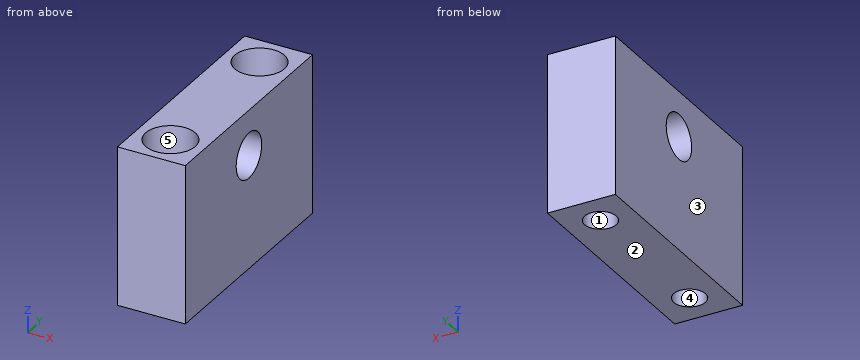
```python
from build123d import *

# Parameters (mm, degrees)
F0_W     = 15
F0_H     = 50
F1_DEPTH = 35
F2_R     = 5
F3_DEPTH = 15
F4_R     = 3.5
F5_DEPTH = 35
F6_R     = 5.5
F7_DEPTH = 9.5


with BuildPart() as f1:
    # F0 (on Top) → F1 (new body)
    with BuildSketch(Plane.XY):
        Rectangle(F0_W, F0_H)
    extrude(amount=F1_DEPTH)

    # F2 (on face) → F3 (cut, through all)
    with BuildSketch(Plane.YZ.offset(7.5)):
        with Locations((0, 25)):
            Circle(F2_R)
    extrude(amount=-F3_DEPTH, mode=Mode.SUBTRACT)

    # F4 (on face) → F5 (cut, through all)
    with BuildSketch(Plane.XY.offset(35)):
        with Locations((0, -17.5)):
            Circle(F4_R)
        with Locations((0, 17.5)):
            Circle(F4_R)
    extrude(amount=-F5_DEPTH, mode=Mode.SUBTRACT)

    # F6 (on face) → F7 (cut)
    with BuildSketch(Plane.XY.offset(35)):
        with Locations((0, -17.5)):
            Circle(F6_R)
        with Locations((0, 17.5)):
            Circle(F6_R)
    extrude(amount=-F7_DEPTH, mode=Mode.SUBTRACT)


solid = f1.part
```
The listing builds one solid part. Answer for the finished solid, in the listing's coordinates (mm). Face numbers are marked on the shaded views. A direction names the side the tool comes from. Round coordinates to 2 decimals unless told otherwise and drop trailing zeros. Loops run counter-clockwise (first coordinate to the right, second up) from the corner with the lowest first, then second, coordinate; pieces in that order, holes last.
1) Given P1, Ø3, axis at y = 2.5, z = 26, coming from the -X side, flat-ended and moving along its own axis, determine where the tip first touches the part or whether it passes through.
Outcome:
P1: passes through
2) A cutting plane is placed at D-D on x = -2.25. Determine the outline of the cut face in (y, z), plus the area to 3 significant figures.
Outcome:
outline: (-25, 0) - (-20.18, 0) - (-20.18, 25.5) - (-22.52, 25.5) - (-22.52, 35) - (-25, 35) - close; (-14.82, 0) - (14.82, 0) - (14.82, 25.5) - (12.48, 25.5) - (12.48, 35) - (-12.48, 35) - (-12.48, 25.5) - (-14.82, 25.5) - close; (20.18, 0) - (25, 0) - (25, 35) - (22.52, 35) - (22.52, 25.5) - (20.18, 25.5) - close; hole circle Ø10 at (0, 25)
area: 1,210 mm2
3) A cutting plane is placed at C-C on z = 9.5. Determine the outline of the cut face in (x, y), plus the area to 3 significant figures.
Outcome:
outline: (-7.5, -25) - (7.5, -25) - (7.5, 25) - (-7.5, 25) - close; hole circle Ø7 at (0, -17.5); hole circle Ø7 at (0, 17.5)
area: 673 mm2
4) Consider line 1 (Y direction, x = 0, z = 31); line 2 (Y direction, x = 5, z = 32); line 3 (Y direction, x = -0.25, z = 26). Determine where each line is inside the solid, lowest interval first.
Outcome:
line 1: y = -25 to -23, -12 to 12, 23 to 25
line 2: y = -25 to -19.79, -15.21 to 15.21, 19.79 to 25
line 3: y = -25 to -22.99, -12.01 to -4.9, 4.9 to 12.01, 22.99 to 25
5) A cutting plane is placed at A-A on y = 17.5. Determine the outline of the cut face in (x, z), plus the area to 3 significant figures.
Outcome:
outline: (-7.5, 0) - (-3.5, 0) - (-3.5, 25.5) - (-5.5, 25.5) - (-5.5, 35) - (-7.5, 35) - close; (3.5, 0) - (7.5, 0) - (7.5, 35) - (5.5, 35) - (5.5, 25.5) - (3.5, 25.5) - close
area: 242 mm2
6) For the marked faces 4 and 5, determine the directions among +Z, -Z, +X, -X, +Y, -Y from which every point of the face is accessible in a straight line to the end or side of a thin tool.
Outcome:
face 4: +Z, -Z
face 5: +Z
7) For a pull along X with two mould halves and no side action, classify the marked faces 1, 2 and 3 as released by +X, released by -X, zero draft, split by the parting line, or undercut.
Outcome:
face 1: undercut
face 2: zero draft
face 3: released by -X
8) A cutting plane is placed at B-B on x = 0. Determine the outline of the cut face in (y, z).
Outcome:
outline: (-25, 0) - (-21, 0) - (-21, 25.5) - (-23, 25.5) - (-23, 35) - (-25, 35) - close; (-14, 0) - (14, 0) - (14, 25.5) - (12, 25.5) - (12, 35) - (-12, 35) - (-12, 25.5) - (-14, 25.5) - close; (21, 0) - (25, 0) - (25, 35) - (23, 35) - (23, 25.5) - (21, 25.5) - close; hole circle Ø10 at (0, 25)
